Model file for the job. Use its own axes, mm. A direction names the side the tool comes from. Coordinates: 2 decimals unless noted, no trailing zeros. Write each loop counter-clockwise with the first axis right and the second up, starting at its lowest first coordinate (ties: lowest second). Pieces come first, ordered by that corner, then holes. Notation, with made-up numbers: (60.25, 41.25) - (98.25, 41.25) arc R21 ccw to (98.25, 79.25) - close; hole circle Ø3 at (67, 40). An arc over 180 degrees is marked (long way). Put each result on its own line as item: value. Start each with the question number.
1. Drill centre lines: L1, parallel to X at y = -3.75, z = 0 (3 decimals); L2, parallel to X at y = -1.65, z = 0 (3 decimals); L3, parallel to Z at x = -38.1, y = -0.85 (3 decimals). Where is each one in solid material? Low to high. Write a range as from..to.
2. Saw through at C-C, the plane y = 4. Write the cut outline in (x, z) (3 decimals).
3. Pull direction X, two halves, no side cores. Call faces 1 (the face through (-60.325, 0, 0)), 2 (the face through (35.57, -6.08, -0.33)), 3 (the face through (0, 10.16, 27)): released by +X, released by -X, zero draft, split by the parting line, or undercut.
4. Saw through at A-A, the plane x = -38.1. Write the cut outline in (y, z) (3 decimals).
5. Which spindle directions (+Z, -Z, +X, -X, +Y, -Y) get a long thin tool onto all of the face, cutting with end or side? Do faces 4 (the face through (-8.84, -5.01, -59.6)), 5 (the face through (-50.8, 5, 0)), 6 (the face through (-8.76, 5.15, -59.6)), 7 (the face through (8.84, 5.01, -59.6)), 8 (the face through (-8.84, 5.01, 59.6)). Say none if no direction does.
6. Drop flat-ended pins along their axis: P1, Ø8, axis at x = -9, z = -18, coming from the +Y side; P2, Ø10, axis at x = -29.5, y = -0.5, coming from the +Z side (3 decimals); P3, Ø6.5, axis at x = -38.1, z = 0, coming from the -Y side (3 decimals); P4, Ø13, axis at x = -38.1, z = 0, coming from the +Y side. Give the stop position or say it passes through.
7. Saw through at D-D, the plane x = 45. Write the cut outline in (y, z) (3 decimals), plus the area to 3 significant figures.
8. Saw through at B-B, the plane z = 0. Write the cut outline in (x, y) (3 decimals).
Autodesk Inventor part; units mm, degrees
ref_plane "YZ Plane" through (0, 0, 0) normal (1, 0, 0) x (0, 1, 0)
ref_plane "XZ Plane" through (0, 0, 0) normal (0, 1, 0) x (-1, 0, 0)
sketch "Sketch1" plane through (0, 0, 0) normal (0, 1, 0) x (-1, 0, 0)
  line L0 (50.8, 21.59) -> (-50.8, 21.59)
  line L1 (-50.8, 21.59) -> (-50.8, -21.59)
  line L2 (-50.8, -21.59) -> (50.8, -21.59)
  line L3 (50.8, -21.59) -> (50.8, 21.59)
  line L4 (50.8, 21.59) -> (-50.8, -21.59) construction
  line L5 (-50.8, 21.59) -> (50.8, -21.59) construction
  line L6 (60.325, 31.115) -> (-60.325, 31.115)
  line L7 (-60.325, 31.115) -> (-60.325, -31.115)
  line L8 (-60.325, -31.115) -> (60.325, -31.115)
  line L9 (60.325, -31.115) -> (60.325, 31.115)
  line L10 (60.325, 31.115) -> (-60.325, -31.115) construction
  line L11 (-60.325, 31.115) -> (60.325, -31.115) construction
  point P0 (0, 0)
extrude "Extrusion1" add sketch "Sketch1" against normal blind 9.525 contours L3 L2 L1 L0 | L9 L8 L7 L6
extrude "Extrusion2" add sketch "Sketch1" along normal blind 10.16
sketch "Sketch5" plane through (0, 0, 0) normal (0, 1, 0) x (1, 0, 0)
  line L0 (-50.8, 21.59) -> (-50.8, -21.59)
  line L1 (50.8, -21.59) -> (50.8, 21.59)
  point P0 (0, 0)
  point P1 (-38.1, 0)
  point P2 (38.1, 0)
  dimension "postHoleCenter" = 12.7
  dimension "d16" = 12.7
hole "Hole1" at (-38.1, 0, 0) at (38.1, 0, 0) direction (0, -1, 0) diameter 5.1054 end through all counterbore diameter 10.16 counterbore depth 2.54
sketch "Sketch6" plane through (-60.325, -9.525, 31.115) normal (0, 0, 1) x (1, 0, 0)
  line L0 (0, 19.685) -> (120.65, 19.685)
  line L1 (66.1909, 19.685) -> (72.0568, 9.525)
  line L2 (72.0568, 9.525) -> (66.1909, -0.635)
  line L3 (66.1909, -0.635) -> (54.4591, -0.635)
  line L4 (54.4591, -0.635) -> (48.5932, 9.525)
  line L5 (48.5932, 9.525) -> (54.4591, 19.685)
  line L6 (54.4591, 19.685) -> (66.1909, 19.685)
  point P0 (60.325, 9.525)
  point P1 (60.325, 9.525)
extrude "Extrusion5" add sketch "Sketch6" along normal blind 57.785
mirror "Mirror2" about plane through (0, 0, 0) normal (0, 0, 1) of "Extrusion5"
equation "\"d4\" = wallThickness"
equation "\"d25\" = hexExtensionLength"
equation "\"wallThickness\" = 9.525"
equation "\"outerWidth\" = innerWidth + 2 * wallThickness"
equation "\"outerLength\" = innerLength + 2 * wallThickness"
equation "\"outerHeight\" = innerDepth + wallThickness"
equation "\"shortenForTestPrint\" = 76.2"
equation "\"hexExtensionLength\" = -0.5 * outerWidth + 0.5 * maxWidth"
equation "\"maxWidth\" = 177.8"
properties part number "connectorToTubeBracketWithHexShaft"
Final values:
1. L1: x = -60.325..-40.653, -35.547..35.547, 40.653..60.325
1. L2: x = -60.325..-43.18, -33.02..33.02, 43.18..60.325
1. L3: z = -31.115..-5.08, 5.08..31.115
2. outline: (-60.325, -31.115) - (-9.422, -31.115) - (-9.422, -88.9) - (9.422, -88.9) - (9.422, -31.115) - (60.325, -31.115) - (60.325, 31.115) - (9.422, 31.115) - (9.422, 88.9) - (-9.422, 88.9) - (-9.422, 31.115) - (-60.325, 31.115) - close; hole (-50.8, -21.59) - (50.8, -21.59) - (50.8, 21.59) - (-50.8, 21.59) - close
3. face 1: released by -X
3. face 2: undercut
3. face 3: zero draft
4. outline: (-9.525, -31.115) - (10.16, -31.115) - (10.16, -21.59) - (0, -21.59) - (0, -5.08) - (-2.54, -5.08) - (-2.54, -2.553) - (-9.525, -2.553) - close; (-9.525, 2.553) - (-2.54, 2.553) - (-2.54, 5.08) - (0, 5.08) - (0, 21.59) - (10.16, 21.59) - (10.16, 31.115) - (-9.525, 31.115) - close
5. face 4: -Z, -X, -Y
5. face 5: +Y
5. face 6: -Z, -X, +Y
5. face 7: -Z, +X, +Y
5. face 8: +Z, -X, +Y
6. P1: stops at y = 10.16
6. P2: stops at z = 31.115
6. P3: stops at y = -9.525
6. P4: stops at y = 0
7. outline: (-9.525, -31.115) - (10.16, -31.115) - (10.16, -21.59) - (0, -21.59) - (0, 21.59) - (10.16, 21.59) - (10.16, 31.115) - (-9.525, 31.115) - close
7. area: 786 mm²
8. outline: (-60.325, -9.525) - (-40.653, -9.525) - (-40.653, -2.54) - (-43.18, -2.54) - (-43.18, 0) - (-50.8, 0) - (-50.8, 10.16) - (-60.325, 10.16) - close; (-35.547, -9.525) - (35.547, -9.525) - (35.547, -2.54) - (33.02, -2.54) - (33.02, 0) - (-33.02, 0) - (-33.02, -2.54) - (-35.547, -2.54) - close; (40.653, -9.525) - (60.325, -9.525) - (60.325, 10.16) - (50.8, 10.16) - (50.8, 0) - (43.18, 0) - (43.18, -2.54) - (40.653, -2.54) - close
